Build history of the part. All positions in model axes, mm. A direction names the side the tool comes from. Give positions to 0.01 mm unless a question says otherwise; leave off trailing zeros. Order: outer loops, then holes, each group sorted by start corner. A loop starts at its lowest first (then second) coordinate and runs counter-clockwise, first axis right, second up. Notation, with made-up numbers: (76.25, -38) - (129.25, -38) arc R11 ccw to (129.25, -23) - close; hole circle Ø3 at (57, 44). An arc over 180 degrees is marked (long way). One line per item, written item: value.
```python
from build123d import *

# Parameters (mm, degrees)
F0_R          = 8.875
F1_DEPTH      = 3
F1_DEPTH_BACK = 3
F2_R          = 2.99999


# Not quite as in the source:
# - a fillet or chamfer is up to 0.001 mm smaller than in the source, because OpenCascade refuses the exact size


with BuildPart() as f1:
    # F0 (on Front) → F1 (new body, two sides)
    with BuildSketch(Plane.XZ) as f1_sk:
        with BuildLine():
            ThreePointArc((-7.3362328356, 7.3362328741), (1.36e-08, 10.375), (7.3362328548, 7.3362328548))
            Line((7.3362328548, 7.3362328548), (0.4560838739, 14.2163818358))
            Line((0.4560838739, 14.2163818358), (0, 13.7602979619))
            Line((0, 13.7602979619), (-0.4560838739, 14.2163818358))
            Line((-0.4560838739, 14.2163818358), (-7.3362328356, 7.3362328741))
        make_face()
        with BuildLine():
            ThreePointArc((-7.3362328073, -7.3362329024), (-10.375, -2e-08), (-7.3362328356, 7.3362328741))
            Line((-7.3362328356, 7.3362328741), (-14.2163818358, 0.4560838739))
            Line((-14.2163818358, 0.4560838739), (-13.7602979619, 0))
            Line((-13.7602979619, 0), (-14.2163818358, -0.4560838739))
            Line((-14.2163818358, -0.4560838739), (-7.3362328073, -7.3362329024))
        make_face()
        with BuildLine():
            ThreePointArc((7.3362328617, -7.3362328479), (9.5852501517, -3.9703406063), (10.375, 0))
            ThreePointArc((10.375, 0), (9.5852501498, 3.9703406108), (7.3362328548, 7.3362328548))
            ThreePointArc((7.3362328548, 7.3362328548), (1.36e-08, 10.375), (-7.3362328356, 7.3362328741))
            ThreePointArc((-7.3362328356, 7.3362328741), (-10.375, -2e-08), (-7.3362328073, -7.3362329024))
            ThreePointArc((-7.3362328073, -7.3362329024), (3.85e-08, -10.375), (7.3362328617, -7.3362328479))
        make_face()
        Circle(F0_R, mode=Mode.SUBTRACT)
        with BuildLine():
            ThreePointArc((7.3362328548, 7.3362328548), (9.5852501498, 3.9703406108), (10.375, 0))
            ThreePointArc((10.375, 0), (9.5852501517, -3.9703406063), (7.3362328617, -7.3362328479))
            Line((7.3362328617, -7.3362328479), (14.2163818358, -0.4560838739))
            Line((14.2163818358, -0.4560838739), (13.7602979619, 0))
            Line((13.7602979619, 0), (14.2163818358, 0.4560838739))
            Line((14.2163818358, 0.4560838739), (7.3362328548, 7.3362328548))
        make_face()
        with BuildLine():
            Line((0.4560838739, -14.2163818358), (7.3362328617, -7.3362328479))
            ThreePointArc((7.3362328617, -7.3362328479), (3.85e-08, -10.375), (-7.3362328073, -7.3362329024))
            Line((-7.3362328073, -7.3362329024), (-0.4560838739, -14.2163818358))
            Line((-0.4560838739, -14.2163818358), (0, -13.7602979619))
            Line((0, -13.7602979619), (0.4560838739, -14.2163818358))
        make_face()
    extrude(amount=F1_DEPTH)
    extrude(f1_sk.sketch, amount=-F1_DEPTH_BACK)

    # F2 (radius 3 in the source; OpenCascade refuses exactly that, so slightly less here)
    f2_edges = [f1.edges().sort_by_distance(p)[0] for p in [
        (0.228042, -3, 13.98834),
        (-0.228042, -3, 13.98834),
        (13.98834, -3, 0.228042),
        (13.98834, -3, -0.228042),
        (0.228042, -3, -13.98834),
        (-0.228042, -3, -13.98834),
        (-13.98834, -3, 0.228042),
        (-13.98834, -3, -0.228042),
        (-13.98834, 3, 0.228042),
        (-13.98834, 3, -0.228042),
        (-0.228042, 3, -13.98834),
        (0.228042, 3, -13.98834),
        (13.98834, 3, 0.228042),
        (13.98834, 3, -0.228042),
        (0.228042, 3, 13.98834),
        (-0.228042, 3, 13.98834),
    ]]
    fillet(f2_edges, radius=F2_R)


solid = f1.part
```
(1) Drill centre lines: line 1 (Z direction, x = -7, y = -2); line 2 (X direction, y = -2.25, z = -4). Where is each one in solid material? Low to high.
Completed:
line 1: -7.67 to -5.46, 5.46 to 7.67
line 2: -10.67 to -7.92, 7.92 to 10.67
(2) 3-axis set-ups, long thin cutter, end or side, ignore diameter. For faces 4 (the face through (-12.63, -2.44, -0.64)), 5 (the face through (0.646, -2.476, 12.559)), 6 (the face through (12.63, -2.44, 0.64)), 7 (the face through (-0.64, 2.44, 12.63)), 8 (the face through (-12.6, 2.44, 0.61)): which of +Z, -Z, +X, -X, +Y, -Y reach the whole face in a straight line?
Completed:
face 4: -X, -Y
face 5: +Z, -Y
face 6: +X, -Y
face 7: +Z, +Y
face 8: -X, +Y
(3) Slice it at D-D, the plane y = -0.75. Give the cut face in (x, z) (3 decimals).
Completed:
outline: (-14.149, -0.523) - (-0.523, -14.149) - (0, -13.626) - (0.523, -14.149) - (14.149, -0.523) - (13.626, 0) - (14.149, 0.523) - (0.523, 14.149) - (0, 13.626) - (-0.523, 14.149) - (-14.149, 0.523) - (-13.626, 0) - close; hole circle Ø17.75 at (0, 0)
(4) Slice it at C-C, the plane y = -2.25. Give the cut face in (x, z) (3 decimals), and give its area (3 significant figures).
Completed:
outline: (-13.498, -1.174) - (-1.174, -13.498) - (0, -12.324) - (1.174, -13.498) - (13.498, -1.174) - (12.324, 0) - (13.498, 1.174) - (1.174, 13.498) - (0, 12.324) - (-1.174, 13.498) - (-13.498, 1.174) - (-12.324, 0) - close; hole circle Ø17.75 at (0, 0)
area: 172 mm²
(5) Slice it at A-A, the plane z = 5. Give the cut face in (x, y), and give its area (3 significant figures).
Completed:
outline: (-9.67, -3) - (-7.33, -3) - (-7.33, 3) - (-9.67, 3) - close; (7.33, -3) - (9.67, -3) - (9.67, 3) - (7.33, 3) - close
area: 28.1 mm²
(6) Pull direction X, two halves, no side cores. Call faces 1 (the face through (0.64, 2.44, -12.63)), 2 (the face through (-1, -3, 9)), 3 (the face through (12.6, 2.44, -0.61)): +X half, -X half, draft (parallel to the pull), parting line (faces both ways), or undercut.
Completed:
face 1: undercut
face 2: draft
face 3: +X half
(7) Pin check, flat tips, straight feed: P1, Ø3, axis at y = 1, z = -4, coming from the +X side; P2, Ø2, axis at x = 8, y = 1.5, coming from the -Z side. Stop position of each tip, or through.
Completed:
P1: x = 12.17
P2: z = -7.67
(8) Slice it at B-B, the plane x = -8. Give the cut face in (y, z), and give its area (3 significant figures).
Completed:
outline: (-3, -6.67) - (3, -6.67) - (3, -3.84) - (-3, -3.84) - close; (-3, 3.84) - (3, 3.84) - (3, 6.67) - (-3, 6.67) - close
area: 34.0 mm²
